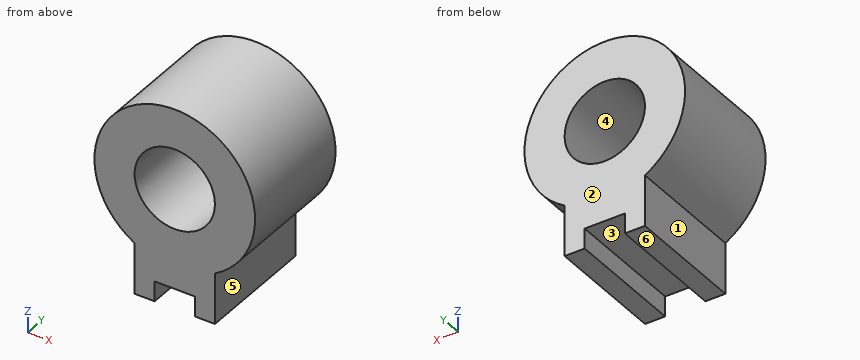
```python
from build123d import *

# Parameters (mm, degrees)
F0_R     = 20
F1_DEPTH = 60


with BuildPart() as f1:
    # F0 (on Front) → F1 (new body)
    with BuildSketch(Plane.XZ):
        with BuildLine():
            Line((-51.450498, -23.447088), (-51.450498, -43.447088))
            Line((-51.450498, -43.447088), (-41.450498, -43.447088))
            Line((-41.450498, -43.447088), (-41.450498, -33.447088))
            Line((-41.450498, -33.447088), (-21.450498, -33.447088))
            Line((-21.450498, -33.447088), (-21.450498, -43.447088))
            Line((-21.450498, -43.447088), (-11.450498, -43.447088))
            Line((-11.450498, -43.447088), (-11.450498, -23.447088))
            Line((-11.450498, -23.447088), (-11.450498, -18.088088))
            ThreePointArc((-11.450498, -18.088088), (-31.450498, 56.552928), (-51.450498, -18.088088))
            Line((-51.450498, -18.088088), (-51.450498, -23.447088))
        make_face()
        with Locations((-31.450498, 16.552928)):
            Circle(F0_R, mode=Mode.SUBTRACT)
    extrude(amount=F1_DEPTH)


solid = f1.part
```
Could you check a few things on this model? Use its own coordinates, in mm. Face numbers are marked on the shaded views. A direction names the side the tool comes from. Coordinates: 2 decimals unless noted, no trailing zeros. Loops run counter-clockwise (first coordinate to the right, second up) from the corner with the lowest first, then second, coordinate; pieces in that order, holes last.
1) Please list where these lines run through material, in increasing order: line 1 along X through (y, z) = (-29, -34); line 2 along Z through (x, y) = (-19.5, -24); line 3 along X through (y, z) = (-17, 2.5).
Reported:
line 1: x = -51.45 to -41.45, -21.45 to -11.45
line 2: z = -43.45 to 0.52, 32.59 to 54.73
line 3: x = -68.9 to -45.68, -17.22 to 6
2) Imagine slicing it at B-B (x = -29). List the corners of the cut face in (y, z) for me, and give its area (3 significant figures).
Reported:
outline: (-60, -33.45) - (0, -33.45) - (0, -3.3) - (-60, -3.3) - close; (-60, 36.4) - (0, 36.4) - (0, 56.48) - (-60, 56.48) - close
area: 3,010 mm2
3) Imagine slicing it at A-A (z = 3). List the corners of the cut face in (x, y) for me.
Reported:
outline: (-69.08, -60) - (-46.16, -60) - (-46.16, 0) - (-69.08, 0) - close; (-16.74, -60) - (6.18, -60) - (6.18, 0) - (-16.74, 0) - close
4) Imagine slicing it at D-D (z = -27.5). List the corners of the cut face in (x, y) for me, and give its area (3 significant figures).
Reported:
outline: (-51.45, -60) - (-11.45, -60) - (-11.45, 0) - (-51.45, 0) - close
area: 2,400 mm2
5) Which directions (+Z, -Z, +X, -X, +Y, -Y) give clear straight access to the entire face, cutting with the end or side of a thin tool? Please do the marked faces 1, 2 and 3.
Reported:
face 1: -Z, -X, +Y, -Y
face 2: +Z, -Z, +X, -X, +Y
face 3: -Z, +Y, -Y
6) Will these pins go through, and if not, where does the flat tip stop? pin 1 Ø3 at (y, z) = (-29.5, -40.5) entering from -X; pin 2 Ø20.5 at (y, z) = (-41.5, -36) entering from +X; pin 3 Ø4 at (x, y) = (0, -48) entering from -Z.
Reported:
pin 1: stops at x = -51.45
pin 2: stops at x = -11.45
pin 3: stops at z = -10.51
7) Imagine slicing it at C-C (y = -41.5). List the corners of the cut face in (x, z) for me, and give its area (3 significant figures).
Reported:
outline: (-51.45, -43.45) - (-41.45, -43.45) - (-41.45, -33.45) - (-21.45, -33.45) - (-21.45, -43.45) - (-11.45, -43.45) - (-11.45, -18.09) arc R40 ccw (long way) to (-51.45, -18.09) - close; hole circle Ø40 at (-31.45, 16.55)
area: 4,440 mm2
8) Thinking about a two-plate mould opening in X: for the marked faces 4, 5 and 6, which applies, released by +X, released by -X, zero draft, split by the parting line, or undercut?
Reported:
face 4: undercut
face 5: released by +X
face 6: zero draft
